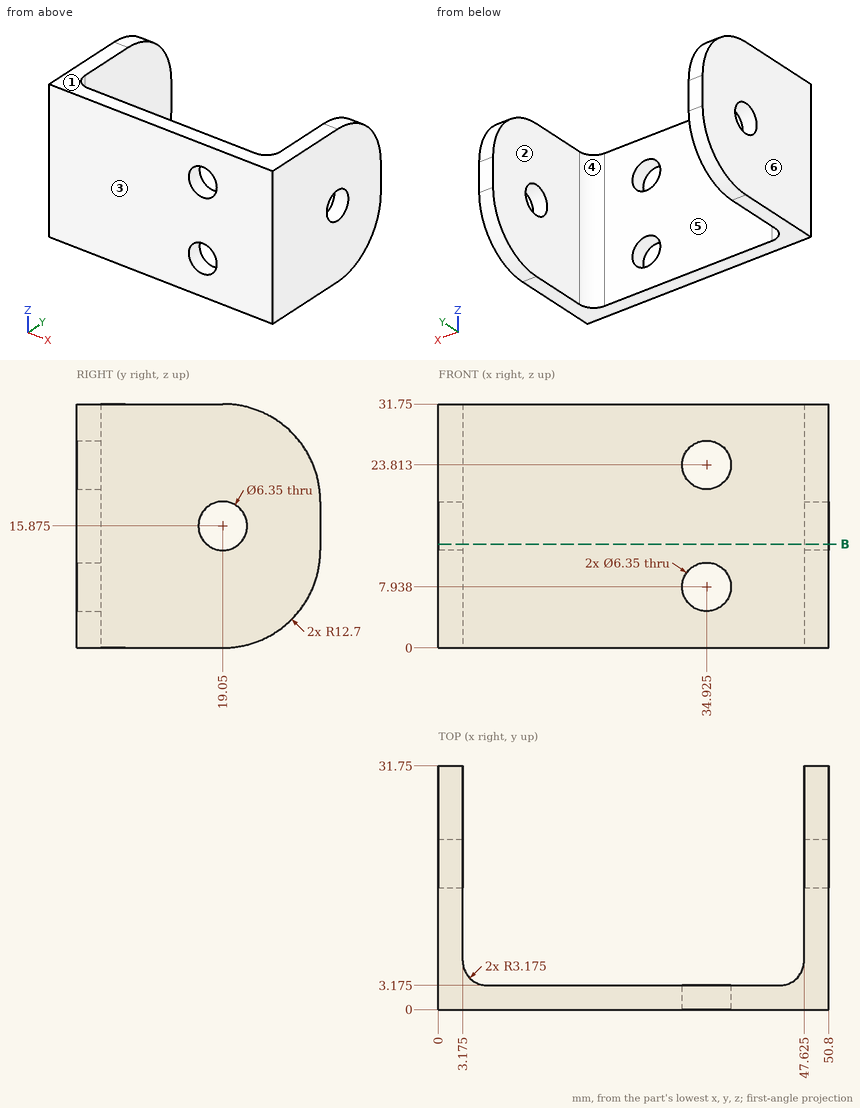
Print and shaded views of the part. All mm, measured from the part's lowest x, y and z. A direction names the side the tool comes from. Coordinates: 2 decimals unless noted, no trailing zeros. Return JSON: item names as keys, results as strings.
1. 3-axis set-ups, long thin cutter, end or side, ignore diameter. For the marked faces 1 and 2: which of +Z, -Z, +X, -X, +Y, -Y reach the whole face in a straight line?
Determined:
{"face 1": "+Z, +X, -X, +Y, -Y", "face 2": "+Z, -Z, +Y"}
2. Pull direction X, two halves, no side cores. Call the marked faces 3, 4, 5 and 6: pulls with the +X half, pulls with the -X half, needs draft (parallel to the pull), parting line crosses it, or undercut.
Determined:
{"face 3": "needs draft", "face 4": "undercut", "face 5": "undercut", "face 6": "pulls with the -X half"}
3. Probe L1, parallel to X at y = 26.5, z = 19.5 (1 decimal); L2, parallel to Z at x = 1, y = 19; L3, parallel to Y at x = 17, z = 6 (1 decimal). List the from-to ranges inside material, lowest first.
Determined:
{"L1": "0 to 3.2, 47.6 to 50.8", "L2": "0 to 12.7, 19.05 to 31.75", "L3": "0 to 3.2"}
4. Flat gauge pin, fed straight in: pin 1 Ø9.5 at (x, z) = (29.5, 10.5) entering from +Y (1 decimal). Where does the tip first touch, or does it go through?
Determined:
{"pin 1": "y = 3.2"}
5. Saw through at B-B, the plane z = 13.5. Count the separate pieces of the cut face and the enclosed holes in it.
Determined:
{"separate pieces": "3", "enclosed holes": "0"}
